Here's the drawing with two shaded views (mm, measured from the low corner). I have some questions. A direction names the side the tool comes from. Coordinates: 2 decimals unless noted, no trailing zeros. Loops run counter-clockwise (first coordinate to the right, second up) from the corner with the lowest first, then second, coordinate; pieces in that order, holes last. Notation, with made-up numbers: (-29.5, 5) - (-4.5, 5) arc R14 ccw to (-4.5, 24) - close; hole circle Ø10 at (-13.75, 61.5). An arc over 180 degrees is marked (long way). Use a Markdown table: item, result.
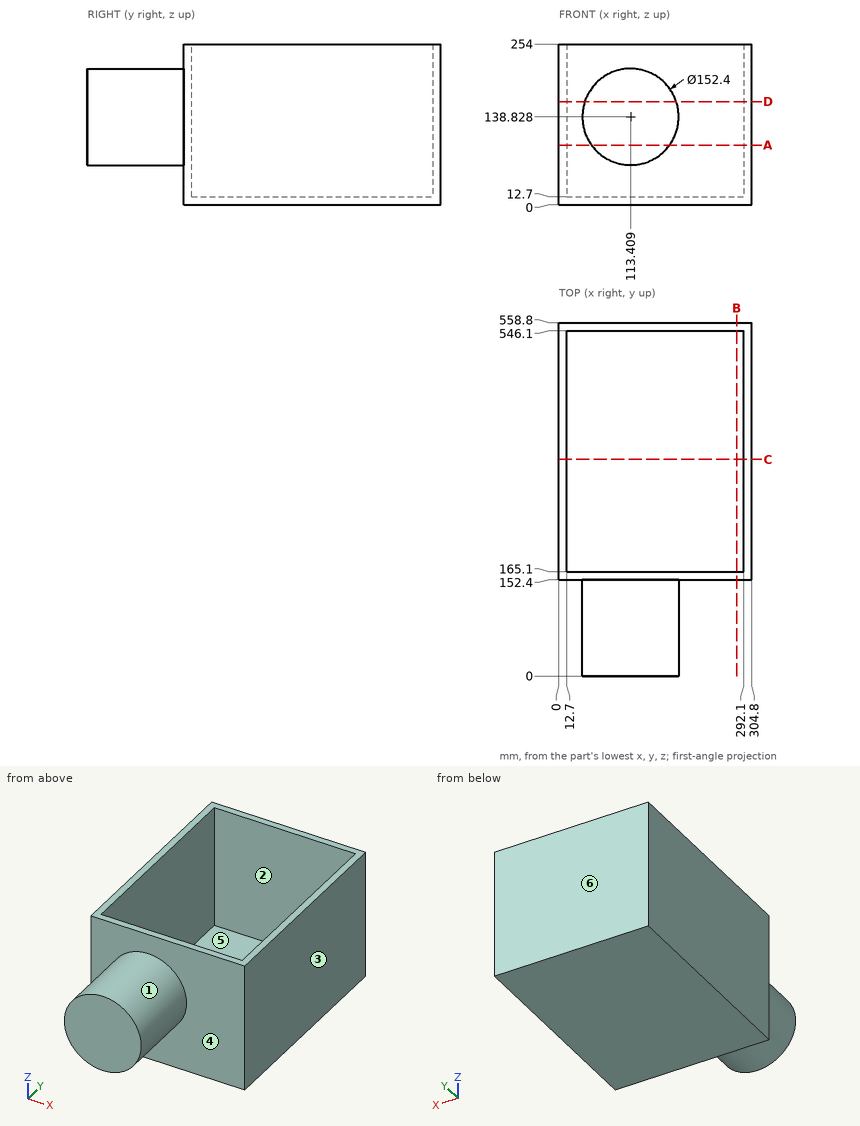
Q1. I want a section at D-D, the plane z = 163. Write out the boundary of the cut face in (x, y) (1 decimal).
Check values:
| item | result |
|---|---|
| outline | (0, 152.4) - (41.1, 152.4) - (41.1, 0) - (185.7, 0) - (185.7, 152.4) - (304.8, 152.4) - (304.8, 558.8) - (0, 558.8) - close; hole (12.7, 165.1) - (292.1, 165.1) - (292.1, 546.1) - (12.7, 546.1) - close |
Q2. Please list where these lines run through material, in increasing order: L1, parallel to X at y = 474, z = 34.5; L2, parallel to Y at x = 275.5, z = 220.5; L3, parallel to Y at x = 132, z = 106.5. Write a range as from..to.
Check values:
| item | result |
|---|---|
| L1 | 0..12.7, 292.1..304.8 |
| L2 | 152.4..165.1, 546.1..558.8 |
| L3 | 0..165.1, 546.1..558.8 |
Q3. Which directions (+Z, -Z, +X, -X, +Y, -Y) give clear straight access to the entire face, cutting with the end or side of a thin tool? Please do the marked faces 4, 5 and 6.
Check values:
| item | result |
|---|---|
| face 4 | -Y |
| face 5 | +Z |
| face 6 | +Z, -Z, +X, -X, +Y |
Q4. Will this pin go through, and if not, where does the flat tip stop? P1, Ø2, axis at x = 161.5, y = 206, coming from the +Z side.
Check values:
| item | result |
|---|---|
| P1 | z = 12.7 |
Q5. I want a section at A-A, the plane z = 94. Write out the boundary of the cut face in (x, y), then the cut area to 3 significant figures.
Check values:
| item | result |
|---|---|
| outline | (0, 152.4) - (51.79, 152.4) - (51.79, 0) - (175.03, 0) - (175.03, 152.4) - (304.8, 152.4) - (304.8, 558.8) - (0, 558.8) - close; hole (12.7, 165.1) - (292.1, 165.1) - (292.1, 546.1) - (12.7, 546.1) - close |
| area | 36,200 mm^2 |
Q6. If we mould it in two halves opening along X, with no side actions, what happens to the marked faces 1, 2 and 3? For each: pulls with the +X half, pulls with the -X half, needs draft (parallel to the pull), parting line crosses it, or undercut.
Check values:
| item | result |
|---|---|
| face 1 | parting line crosses it |
| face 2 | undercut |
| face 3 | pulls with the +X half |
Q7. I want a section at B-B, the plane x = 281. Write out the boundary of the cut face in (y, z), then the cut area to 3 significant figures.
Check values:
| item | result |
|---|---|
| outline | (152.4, 0) - (558.8, 0) - (558.8, 254) - (546.1, 254) - (546.1, 12.7) - (165.1, 12.7) - (165.1, 254) - (152.4, 254) - close |
| area | 11,300 mm^2 |
Q8. I want a section at C-C, the plane y = 342.5. Write out the boundary of the cut face in (x, z), then the cut area to 4 significant figures.
Check values:
| item | result |
|---|---|
| outline | (0, 0) - (304.8, 0) - (304.8, 254) - (292.1, 254) - (292.1, 12.7) - (12.7, 12.7) - (12.7, 254) - (0, 254) - close |
| area | 10,000 mm^2 |
